Check sheet for the modelled part. Datum: model origin and axes. Units: mm. A direction names the side the tool comes from. Round coordinates to 2 decimals unless told otherwise and drop trailing zeros. Loops run counter-clockwise (first coordinate to the right, second up) from the corner with the lowest first, then second, coordinate; pieces in that order, holes last. Notation, with made-up numbers: M -19.75,27 L -12.75,27 A31 cw -12.75,62 Z; hole C 17,47.25 d10. An arc over 180 degrees is marked long. One line per question, with ' | ' between items. Start each with the question number.
(1) Section check D-D (z = 24). Record the boundary of the cut face in (x, y).
(2) Tool access check on faces 1 (the face through (19.5, 31.6, 23.7)), 2 (the face through (60, 22, 11)), 3 (the face through (5, 2.5, 11)), 4 (the face through (70, 1, 11)). Record the directions out of +Z, -Z, +X, -X, +Y, -Y that give a thin tool (end or side, any length) a straight path to the whole face; none if there is none.
(3) Section check A-A (z = 13.5). Record the boundary of the cut face in (x, y), and give its area (3 significant figures).
(4) Go/stop test with flat-tipped pins: P1, Ø11, axis at y = 21.5, z = 10, coming from the -X side; P2, Ø2, axis at y = 16, z = 5, coming from the +X side. Record where each tip stops, or that it passes through.
(5) Section check B-B (x = 25). Record the boundary of the cut face in (y, z).
(6) Thickness scan on probe 1 along Z at (x, y) = (40, 10.5); probe 2 along Z at (x, y) = (28.5, 32.5); probe 3 along X at (y, z) = (22, 8.75). Record the ranges inside material, lowest first. Write a range as [from, to].
(7) Section check C-C (y = 26.5). Record the boundary of the cut face in (x, z), and give its area (3 significant figures).
```python
from build123d import *

# Parameters (mm, degrees)
SKETCH1_W           = 70
SKETCH1_H           = 40
BOSS_EXTRUDE1_DEPTH = 22.5
SKETCH2_R           = 7.5
BOSS_EXTRUDE2_DEPTH = 2.5
SKETCH3_R           = 6
BOSS_EXTRUDE3_DEPTH = 2.5
SKETCH4_W           = 22.5
SKETCH4_H           = 37.5
CUT_EXTRUDE1_DEPTH  = 10
SKETCH5_W           = 22.5
SKETCH5_H           = 37.5
CUT_EXTRUDE2_DEPTH  = 10


with BuildPart() as part:
    # Sketch1 → Boss-Extrude1 (new body)
    with BuildSketch(Plane.XY):
        with Locations((35, 20)):
            Rectangle(SKETCH1_W, SKETCH1_H)
    extrude(amount=BOSS_EXTRUDE1_DEPTH)

    # Sketch2 → Boss-Extrude2 (add)
    with BuildSketch(Plane.XY.offset(22.5)):
        with Locations((25, 26.5)):
            Circle(SKETCH2_R)
    extrude(amount=BOSS_EXTRUDE2_DEPTH)

    # Sketch3 → Boss-Extrude3 (add)
    with BuildSketch(Plane.XY.offset(25)):
        with Locations((25, 26.5)):
            Circle(SKETCH3_R)
    extrude(amount=BOSS_EXTRUDE3_DEPTH)

    # Sketch4 → Cut-Extrude1 (cut)
    with BuildSketch(Plane.ZY):
        with Locations((11.25, 21.25)):
            Rectangle(SKETCH4_W, SKETCH4_H)
    extrude(amount=-CUT_EXTRUDE1_DEPTH, mode=Mode.SUBTRACT)

    # Sketch5 → Cut-Extrude2 (cut)
    with BuildSketch(Plane(origin=(70, 0, 0), x_dir=(0, 0, -1), z_dir=(1, 0, 0))):
        with Locations((-11.25, 21.25)):
            Rectangle(SKETCH5_W, SKETCH5_H)
    extrude(amount=-CUT_EXTRUDE2_DEPTH, mode=Mode.SUBTRACT)


solid = part.part
```
The answers:
1) outline: C 25,26.5 d15
2) face 1: +Z | face 2: +Z, -Z, +X, +Y | face 3: +Z, -Z, -X, +Y | face 4: +Z, -Z, +X, +Y, -Y
3) outline: M 0,0 L 70,0 L 70,2.5 L 60,2.5 L 60,40 L 10,40 L 10,2.5 L 0,2.5 Z | area: 2,050 mm²
4) P1: x = 10 | P2: x = 60
5) outline: M 0,0 L 40,0 L 40,22.5 L 34,22.5 L 34,25 L 32.5,25 L 32.5,27.5 L 20.5,27.5 L 20.5,25 L 19,25 L 19,22.5 L 0,22.5 Z
6) probe 1: [0, 22.5] | probe 2: [0, 25] | probe 3: [10, 60]
7) outline: M 10,0 L 60,0 L 60,22.5 L 32.5,22.5 L 32.5,25 L 31,25 L 31,27.5 L 19,27.5 L 19,25 L 17.5,25 L 17.5,22.5 L 10,22.5 Z | area: 1,190 mm²
